```python
from build123d import *

# Parameters (mm, degrees)
F1_DEPTH = 19.05


# Not quite as in the source:
# - a feature of the source that left no trace in its solid (it failed there, or was rolled back) is left out


with BuildPart() as f1:
    # F0 (on Front) → F1 (new body, symmetric)
    with BuildSketch(Plane.XZ):
        with BuildLine():
            Line((-19.05, 50.8), (-19.05, 25.4))
            Line((-19.05, 25.4), (19.05, 25.4))
            Line((19.05, 25.4), (19.05, 50.8))
            ThreePointArc((19.05, 50.8), (26.174342016, 67.9996831179), (43.3740251338, 75.1240251338))
            Line((43.3740251338, 75.1240251338), (68.7740251338, 75.1240251338))
            Line((68.7740251338, 75.1240251338), (68.7740251338, 113.2240251338))
            Line((68.7740251338, 113.2240251338), (43.3740251338, 113.2240251338))
            ThreePointArc((43.3740251338, 113.2240251338), (-0.7664263473, 94.9404514811), (-19.05, 50.8))
        make_face()
        Polygon((-19.05, 25.4), (-25.4, 25.4), (-25.4, -25.4), (25.4, -25.4), (25.4, 25.4), (19.05, 25.4), align=None)
        Polygon((68.7740251338, 119.5740251338), (68.7740251338, 113.2240251338), (68.7740251338, 75.1240251338), (68.7740251338, 68.7740251338), (119.5740251338, 68.7740251338), (119.5740251338, 119.5740251338), align=None)
    extrude(amount=F1_DEPTH, both=True)


solid = f1.part
```
Check sheet for the modelled part. Datum: model origin and axes. Units: mm. A direction names the side the tool comes from. Coordinates: 2 decimals unless noted, no trailing zeros. Order: outer loops, then holes, each group sorted by start corner. A loop starts at its lowest first (then second) coordinate and runs counter-clockwise, first axis right, second up. Notation, with made-up numbers: (72.5, 59.25) -> (106.5, 59.25) arc R9 cw to (106.5, 69.25) -> close; hole circle Ø10 at (27.5, -39.5). An arc over 180 degrees is marked (long way). Write each question's results on one line, items separated by ' | '. Start each with the question number.
1) Section check A-A (y = 0). Enter the section's corners in (x, z).
2) Section check B-B (z = 28). Enter the section's corners in (x, y), and give its area (3 significant figures).
3) Set-up check for faces 1 (the face through (68.774, 0, 116)), 2 (the face through (25.986, -0.267, 67.81)), 3 (the face through (19.05, 0, 38)), 4 (the face through (25.4, 0, 0)): record each of +Z, -Z, +X, -X, +Y, -Y from which the full face is reachable in a straight line by a thin tool's end or side.
4) Material ranges on line 1 along Z through (x, y) = (55.5, 5); line 2 along X through (y, z) = (-4, 41); line 3 along Z through (x, y) = (108.5, 13.5), recorded low to high.
5) Draft check along X on faces 5 (the face through (56, 0, 75.124)), 6 (the face through (-25.4, 0, 0)), 7 (the face through (94, 0, 68.774)), 8 (the face through (68.774, 0, 72)). Enter one of: pulls with the +X half, pulls with the -X half, needs draft (parallel to the pull), parting line crosses it, or undercut.
6) Depth check by flat-ended pin: pin 1 (7.5 mm diameter, centred on x = 58.5, y = -8, fed in from -Z); pin 2 (3 mm diameter, centred on y = -6, z = 70.5, fed in from -X); pin 3 (7.5 mm diameter, centred on y = 7, z = 34.5, fed in from -X); pin 4 (8 mm diameter, centred on x = 22.5, z = 58, fed in from -Y). Enter the tip coordinate at first touch or a pass-through.
7) Section check C-C (x = 49.5). Enter the section's corners in (y, z), and give its area (3 significant figures).
Checked values:
1) outline: (-25.4, -25.4) -> (25.4, -25.4) -> (25.4, 25.4) -> (19.05, 25.4) -> (19.05, 50.8) arc R24.32 cw to (43.37, 75.12) -> (68.77, 75.12) -> (68.77, 68.77) -> (119.57, 68.77) -> (119.57, 119.57) -> (68.77, 119.57) -> (68.77, 113.22) -> (43.37, 113.22) arc R62.42 ccw to (-19.05, 50.8) -> (-19.05, 25.4) -> (-25.4, 25.4) -> close
2) outline: (-19.05, -19.05) -> (19.05, -19.05) -> (19.05, 19.05) -> (-19.05, 19.05) -> close | area: 1,450 mm²
3) face 1: +Z, -X, +Y, -Y | face 2: +Y, -Y | face 3: +X, +Y, -Y | face 4: -Z, +X, +Y, -Y
4) line 1: 75.12 to 113.22 | line 2: -19.05 to 19.05 | line 3: 68.77 to 119.57
5) face 5: undercut | face 6: pulls with the -X half | face 7: needs draft | face 8: undercut
6) pin 1: z = 75.12 | pin 2: x = -16.34 | pin 3: x = -19.05 | pin 4: y = -19.05
7) outline: (-19.05, 75.12) -> (19.05, 75.12) -> (19.05, 113.22) -> (-19.05, 113.22) -> close | area: 1,450 mm²
